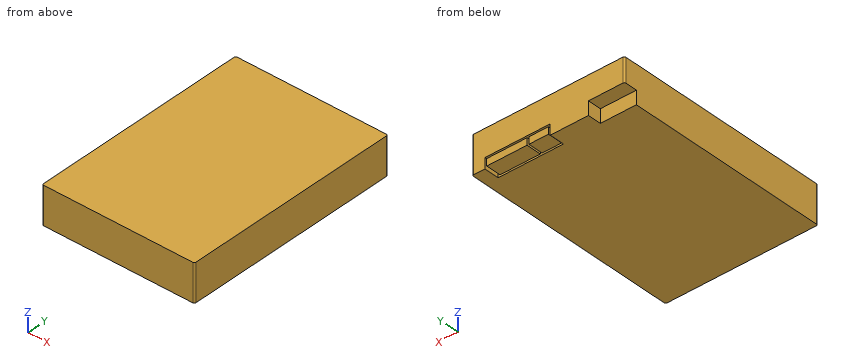
```python
from build123d import *

# Parameters (mm, degrees)
F0_W     = 101.5
F0_H     = 146
F1_DEPTH = 25
F2_W     = 24
F2_H     = 9
F3_DEPTH = 9
F4_R     = 1
F5_W     = 43.5
F5_H     = 7
F6_DEPTH = 10
F7_W     = 26.9
F7_H     = 4.6
F7_W_2   = 13
F8_DEPTH = 10


with BuildPart() as f1:
    # F0 (on Top) → F1 (new body)
    with BuildSketch(Plane.XY):
        Rectangle(F0_W, F0_H)
    extrude(amount=F1_DEPTH)

    # F2 (on face) → F3 (cut)
    with BuildSketch(Plane(origin=(0, 73, 0), x_dir=(-1, 0, 0), z_dir=(0, 1, 0))):
        with Locations((38.75, 4.5)):
            Rectangle(F2_W, F2_H)
    extrude(amount=-F3_DEPTH, mode=Mode.SUBTRACT)

    # F4
    f4_edges = [f1.edges().sort_by_distance(p)[0] for p in [
        (50.75, 73, 12.5),
        (-50.75, 73, 17),
        (-50.75, -73, 12.5),
        (50.75, -73, 12.5),
    ]]
    fillet(f4_edges, radius=F4_R)

    # F5 (on face) → F6 (cut)
    with BuildSketch(Plane(origin=(0, 73, 0), x_dir=(-1, 0, 0), z_dir=(0, 1, 0))):
        with Locations((-20.5, 3.5)):
            Rectangle(F5_W, F5_H)
    extrude(amount=-F6_DEPTH, mode=Mode.SUBTRACT)

    # F7 (on face) → F8 (join)
    with BuildSketch(Plane(origin=(0, 63, 0), x_dir=(-1, 0, 0), z_dir=(0, 1, 0))):
        with Locations((-27.6, 3.5)):
            Rectangle(F7_W, F7_H)
        with Locations((-6.45, 3.5)):
            Rectangle(F7_W_2, F7_H)
    extrude(amount=F8_DEPTH)


solid = f1.part
```
Read the model definition and answer for the solid it produces. Units are mm, in the model's axes. Coordinates: 2 decimals unless noted, no trailing zeros. Loops run counter-clockwise (first coordinate to the right, second up) from the corner with the lowest first, then second, coordinate; pieces in that order, holes last.
(1) Flat-ended cylindrical pins translate along their axes: pin 1 Ø2 at (x, y) = (34.5, 30) entering from -Z; pin 2 Ø2 at (y, z) = (70, 4.5) entering from -X; pin 3 Ø3 at (x, y) = (29.5, 69.5) entering from -Z; pin 4 Ø4.5 at (x, y) = (-35, 69) entering from -Z. Find the tip coordinate at first contact, or state that the pin passes through.
Solution:
pin 1: stops at z = 0
pin 2: stops at x = -26.75
pin 3: stops at z = 1.2
pin 4: stops at z = 9
(2) Consider line 1 along Y through (x, z) = (-31, 7.75). Determine where the line is inside the solid, lowest interval first.
Solution:
line 1: y = -73 to 64
(3) The part is cut by section A-A (z = 4.25). Determine the outline of the cut face in (x, y), and give its area (3 significant figures).
Solution:
outline: (-50.75, -72) arc R1 ccw to (-49.75, -73) - (49.75, -73) arc R1 ccw to (50.75, -72) - (50.75, 72) arc R1 ccw to (49.75, 73) - (42.25, 73) - (42.25, 63) - (41.05, 63) - (41.05, 73) - (14.15, 73) - (14.15, 63) - (12.95, 63) - (12.95, 73) - (-0.05, 73) - (-0.05, 63) - (-1.25, 63) - (-1.25, 73) - (-26.75, 73) - (-26.75, 64) - (-50.75, 64) - close
area: 14,600 mm2
(4) The part is cut by section B-B (x = -40). Determine the outline of the cut face in (y, z).
Solution:
outline: (-73, 0) - (64, 0) - (64, 9) - (73, 9) - (73, 25) - (-73, 25) - close
